```python
from build123d import *

# Parameters (mm, degrees)
SKETCH8_R             = 2.6
SKETCH8_R_2           = 1.1
BOSS_EXTRUDE2_DEPTH   = 5
BOSS_EXTRUDE3_START   = -7.6000001
BOSS_EXTRUDE3_DEPTH   = 7.6000001
BOSS_EXTRUDE3_2_DEPTH = 4
SKETCH10_R            = 1.875
BOSS_EXTRUDE4_DEPTH   = 4.2
SKETCH11_R            = 1
CUT_EXTRUDE1_DEPTH    = 11.524257855


with BuildPart() as part:
    # Sketch8 → Boss-Extrude2 (new body)
    with BuildSketch(Plane.XY):
        Circle(SKETCH8_R)
        Circle(SKETCH8_R_2, mode=Mode.SUBTRACT)
    extrude(amount=BOSS_EXTRUDE2_DEPTH)

    # Boss-Extrude3: read off the stored shape, not the designer's step
    # Boss-Extrude3 outline → Boss-Extrude3 (add)
    with BuildSketch(Plane.XY.offset(BOSS_EXTRUDE3_START)):
        with BuildLine():
            ThreePointArc((0, -2.6), (2.6, 0), (0, 2.6))
            Line((0, 2.6), (0, -2.6))
        make_face()
    extrude(amount=BOSS_EXTRUDE3_DEPTH)

    # Boss-Extrude3 2 outline → Boss-Extrude3 2 (cut)
    with BuildSketch(Plane.YZ):
        with BuildLine():
            Line((2.6, -4), (2.6, -5))
            ThreePointArc((2.6, -5), (1.838477631, -6.838477631), (0, -7.6))
            Line((0, -7.6), (4, -7.6000001))
            Line((4, -7.6000001), (4, -4))
            Line((4, -4), (2.6, -4))
        make_face()
        with BuildLine():
            Line((-4, -7.6000001), (0, -7.6))
            ThreePointArc((0, -7.6), (-1.838477631, -6.838477631), (-2.6, -5))
            Line((-2.6, -5), (-2.6, -4))
            Line((-2.6, -4), (-4, -4))
            Line((-4, -4), (-4, -7.6000001))
        make_face()
    extrude(amount=BOSS_EXTRUDE3_2_DEPTH, mode=Mode.SUBTRACT)

    # Sketch10 → Boss-Extrude4 (add)
    with BuildSketch(Plane.ZY):
        with Locations((-5, 0)):
            Circle(SKETCH10_R)
    extrude(amount=BOSS_EXTRUDE4_DEPTH)

    # Sketch11 → Cut-Extrude1 (cut, through all)
    with BuildSketch(Plane.ZY.offset(4.2)):
        with Locations((-5, 0)):
            Circle(SKETCH11_R)
    extrude(amount=-CUT_EXTRUDE1_DEPTH, mode=Mode.SUBTRACT)


solid = part.part
```
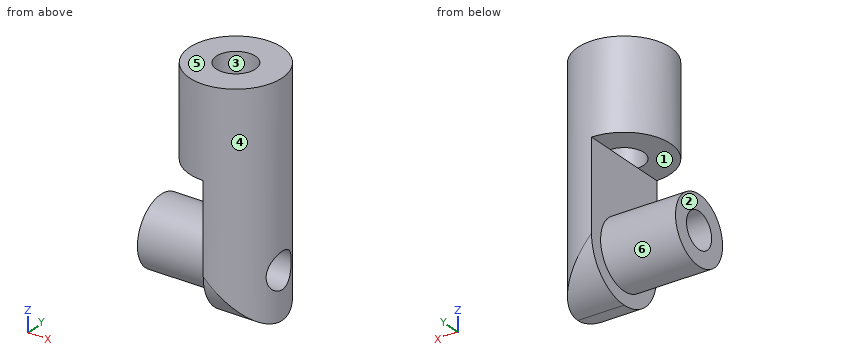
Model file for the job. Use its own axes, mm. Face numbers are marked on the shaded views. A direction names the side the tool comes from. Round coordinates to 2 decimals unless told otherwise and drop trailing zeros. Write each loop counter-clockwise with the first axis right and the second up, starting at its lowest first coordinate (ties: lowest second). Pieces come first, ordered by that corner, then holes. Notation, with made-up numbers: (18.25, -14) - (28.25, -14) arc R28 ccw to (28.25, 11) - close; hole circle Ø2 at (35.5, 37). An arc over 180 degrees is marked (long way). Use CSV: the item, a comma, the result in double quotes. Start each with the question number.
Item 1: Drill centre lines: L1, parallel to Z at x = 1.75, y = 0; L2, parallel to Y at x = 0, z = 3.6. Where is each one in solid material? Low to high. Write a range as [from, to].
Item 2: Band-saw the part on D-D (z = -0.75). Write the cut outline in (x, y).
Item 3: Tool access for the marked faces 1, 2 and 3: list every direction of +Z, -Z, +X, -X, +Y, -Y with a clear straight run to the whole face (end or side of a thin tool).
Item 4: Two-plate mould, pull along Z, no slides. Class the marked faces 4, 5 and 6: released by +Z, released by -Z, zero draft, split by the parting line, or undercut.
Item 5: Band-saw the part on B-B (y = 0.7). Write the cut outline in (x, z).
Item 6: Pin check, flat tips, straight feed: P1, Ø0.6, axis at x = 0.5, y = 0, coming from the +Z side; P2, Ø0.8, axis at x = -1.5, y = -1, coming from the -Z side. Stop position of each tip, or through.
Item 7: Band-saw the part on C-C (x = -1.75). Write the cut outline in (y, z) (3 decimals).
Item 8: Band-saw the part on A-A (x = -0.25). Write the cut outline in (y, z) (3 decimals).
Checked values:
1,L1,"z = [-7.6, -6], [-4, 5]"
1,L2,"y = [-2.6, -1.1], [1.1, 2.6]"
2,outline,"(0, -2.6) arc R2.6 ccw to (0, 2.6) - close"
3,face 1,"-X, +Y, -Y"
3,face 2,"+Z, -Z, -X, +Y, -Y"
3,face 3,"+Z"
4,face 4,"zero draft"
4,face 5,"released by +Z"
4,face 6,"undercut"
5,outline,"(-4.2, -6.74) - (0, -6.74) - (0, -7.5) - (2.5, -7.5) - (2.5, -5.71) - (-4.2, -5.71) - close; (-4.2, -4.29) - (2.5, -4.29) - (2.5, 5) - (0.85, 5) - (0.85, 0) - (0, 0) - (0, -3.26) - (-4.2, -3.26) - close; (-2.5, 0) - (-0.85, 0) - (-0.85, 5) - (-2.5, 5) - close"
6,P1,"stops at z = 0"
6,P2,"stops at z = -6.78"
7,outline,"(-1.923, 0) - (1.923, 0) - (1.923, 5) - (-1.923, 5) - close; circle Ø3.75 at (0, -5); hole circle Ø2 at (0, -5)"
8,outline,"(-2.588, 0) - (-1.071, 0) - (-1.071, 5) - (-2.588, 5) - close; circle Ø3.75 at (0, -5); (1.071, 0) - (2.588, 0) - (2.588, 5) - (1.071, 5) - close; hole circle Ø2 at (0, -5)"
